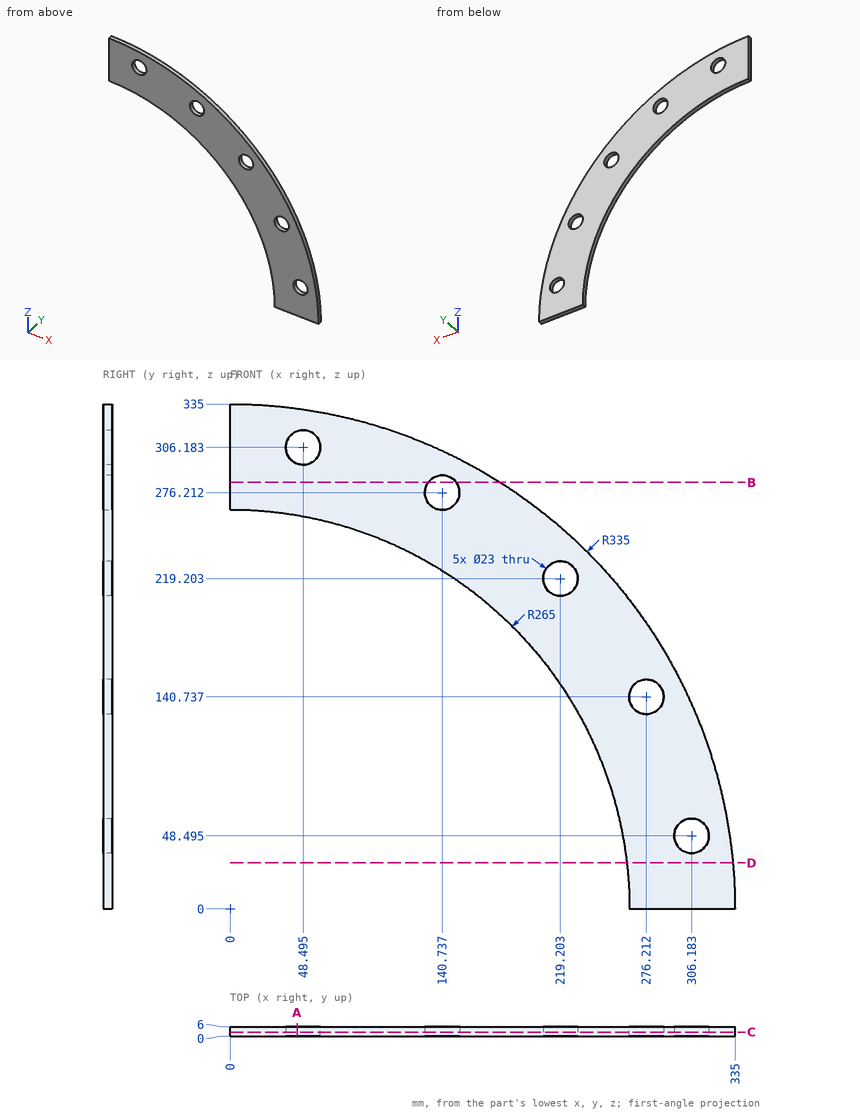
Can you work these out from the drawing? Everything is in mm from the part's minimum corner. Coordinates: 2 decimals unless noted, no trailing zeros. Write each loop counter-clockwise with the first axis right and the second up, starting at its lowest first coordinate (ties: lowest second). Pieces come first, ordered by that corner, then holes. Notation, with made-up numbers: (23, 14.5) -> (46, 14.5) arc R33 cw to (46, 48.5) -> close; hole circle Ø11 at (39, 65). An arc over 180 degrees is marked (long way). Return JSON: item names as keys, results as strings.
(1) Imagine slicing it at D-D, the plane z = 30.5. Please give me the cut outline in (x, y).
Numbers:
{"outline": "(263.24, 0) -> (333.61, 0) -> (333.61, 6) -> (263.24, 6) -> close"}
(2) I'm going to push a flat-ended pin straight in: pin 1 (1.5 mm diameter, centred on x = 202.5, y = 5.5, fed in from -Z). Where does the tip first touch, or does it pass through?
Numbers:
{"pin 1": "stops at z = 170.04"}
(3) Imagine slicing it at A-A, the plane x = 44.5. Please give me the cut outline in (y, z).
Numbers:
{"outline": "(0, 261.24) -> (6, 261.24) -> (6, 295.4) -> (0, 295.4) -> close; (0, 316.97) -> (6, 316.97) -> (6, 332.03) -> (0, 332.03) -> close"}
(4) Imagine slicing it at C-C, the plane y = 2.6. Please give me the cut outline in (x, z) (1 decimal), then the cut area to 3 significant figures.
Numbers:
{"outline": "(0, 265) arc R265 cw to (265, 0) -> (335, 0) arc R335 ccw to (0, 335) -> close; hole circle Ø23 at (48.5, 306.2); hole circle Ø23 at (140.7, 276.2); hole circle Ø23 at (219.2, 219.2); hole circle Ø23 at (276.2, 140.7); hole circle Ø23 at (306.2, 48.5)", "area": "30,900 mm2"}
(5) Imagine slicing it at B-B, the plane z = 283. Please give me the cut outline in (x, y) (1 decimal).
Numbers:
{"outline": "(0, 0) -> (131.5, 0) -> (131.5, 6) -> (0, 6) -> close; (150, 0) -> (179.3, 0) -> (179.3, 6) -> (150, 6) -> close"}
(6) I need wall thicknesses on L1, parallel to Z at x = 148.5, y = 5.4 (1 decimal); L2, parallel to X at y = 2.45, z = 146 (1 decimal); L3, parallel to Z at x = 234, y = 3.05 (1 decimal). Which ranges of each line are inside material? Lowest first, please.
Numbers:
{"L1": "z = 219.5 to 267.7, 284.7 to 300.3", "L2": "x = 221.2 to 266, 286.4 to 301.5", "L3": "z = 124.4 to 239.7"}
